For this review, use the dimensioned drawing (mm, ordinates from the lowest corner) and the shaded views. Round coordinates to 2 decimals unless told otherwise and drop trailing zeros. Loops run counter-clockwise (first coordinate to the right, second up) from the corner with the lowest first, then second, coordinate; pieces in that order, holes last. Notation, with made-up numbers: M 88.25,-28 L 117.25,-28 A30 cw 117.25,1 Z; hole C -20.5,71 d3. An arc over 180 degrees is marked long. Answer as a JSON object with one key per item and string values. Group by question number.
Item 1: Consider section B-B (x = 12.7). Give the boundary of the cut face in (y, z).
Item 2: Consider section D-D (y = 6.35). Give the boundary of the cut face in (x, z).
Item 3: To check wall thickness, follow line 1 (Y direction, x = 19.05, z = 2.5); line 2 (X direction, y = 25.5, z = 1.5); line 3 (Y direction, x = 17.5, z = 5.75). State the ranges of each line that lie inside material, in increasing order.
Item 4: Consider section A-A (y = 31.75). Give the boundary of the cut face in (x, z), and give its area (3 significant figures).
Item 5: Insertion check: P1, Ø3.5, axis at x = 12.7, y = 31.75, coming from the -Z side (3 decimals). The pin has a flat end and moves straight along its axis. Give the tip position at first contact, or say it passes through.
Item 6: The part is to be moulded in two halves that separate along Y. For the marked faces 1, 2 and 3, say which applies: +Y half, -Y half, draft (parallel to the pull), parting line (faces both ways), or undercut.
Item 7: Consider section C-C (z = 2). State how many separate pieces and enclosed holes the cut face has.
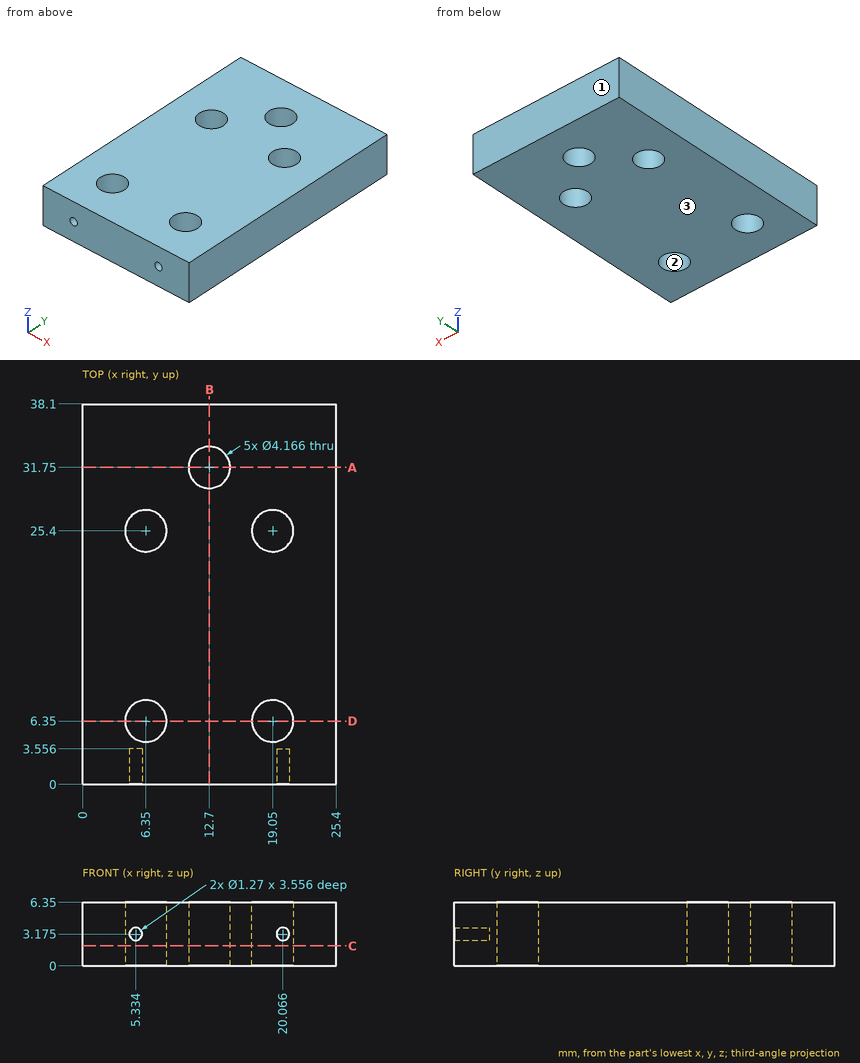
Geometry results:
{
 "1": {"outline": "M 0,0 L 29.67,0 L 29.67,6.35 L 0,6.35 Z; M 33.83,0 L 38.1,0 L 38.1,6.35 L 33.83,6.35 Z"},
 "2": {"outline": "M 0,0 L 4.27,0 L 4.27,6.35 L 0,6.35 Z; M 8.43,0 L 16.97,0 L 16.97,6.35 L 8.43,6.35 Z; M 21.13,0 L 25.4,0 L 25.4,6.35 L 21.13,6.35 Z"},
 "3": {"line 1": "y = 0 to 4.27, 8.43 to 23.32, 27.48 to 38.1", "line 2": "x = 0 to 4.27, 8.43 to 16.97, 21.13 to 25.4", "line 3": "y = 0 to 4.96, 7.74 to 24.01, 26.79 to 38.1"},
 "4": {"outline": "M 0,0 L 10.62,0 L 10.62,6.35 L 0,6.35 Z; M 14.78,0 L 25.4,0 L 25.4,6.35 L 14.78,6.35 Z", "area": "135 mm^2"},
 "5": {"P1": "passes through"},
 "6": {"face 1": "+Y half", "face 2": "undercut", "face 3": "draft"},
 "7": {"separate pieces": "1", "enclosed holes": "5"}
}
